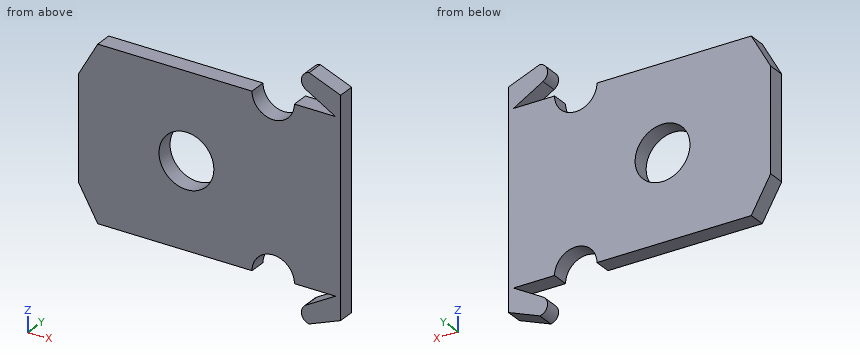
```python
from build123d import *

# Parameters (mm, degrees)
SKETCH1_R           = 0.8
BOSS_EXTRUDE1_DEPTH = 0.5


with BuildPart() as part:
    # Sketch1 → Boss-Extrude1 (new body)
    with BuildSketch(Plane(origin=(0, 0, 0), x_dir=(1, 0, 0), z_dir=(0, 1, 0))):
        with BuildLine():
            Line((0, 1.5), (0, -1.5))
            Line((0, -1.5), (0.566386859, -2.5))
            Line((0.566386859, -2.5), (5.066386859, -2.5))
            ThreePointArc((5.066386859, -2.5), (5.684410747, -1.881976112), (6.302434635, -2.5))
            Line((6.302434635, -2.5), (7.502434635, -2.5))
            Line((7.502434635, -2.5), (6.640167687, -3.000108496))
            ThreePointArc((6.640167687, -3.000108496), (6.510535737, -3.282386176), (6.733125956, -3.499039646))
            Line((6.733125956, -3.499039646), (7.651443218, -3.137476564))
            Line((7.651443218, -3.137476564), (7.651443218, 3.137476564))
            Line((7.651443218, 3.137476564), (6.733125956, 3.499039646))
            ThreePointArc((6.733125956, 3.499039646), (6.510535737, 3.282386176), (6.640167687, 3.000108496))
            Line((6.640167687, 3.000108496), (7.502434635, 2.5))
            Line((7.502434635, 2.5), (6.302434635, 2.5))
            ThreePointArc((6.302434635, 2.5), (5.684410747, 1.881976112), (5.066386859, 2.5))
            Line((5.066386859, 2.5), (0.566386859, 2.5))
            Line((0.566386859, 2.5), (0, 1.5))
        make_face()
        with Locations(Location((3.153366843, 0, 0), (0, 0, 270))):
            Circle(SKETCH1_R, mode=Mode.SUBTRACT)
    extrude(amount=BOSS_EXTRUDE1_DEPTH)


solid = part.part
```
Input: part model. Units: mm. Frame: model coordinates. Give positions to 0.01 mm unless a question says otherwise; leave off trailing zeros. Order: outer loops, then holes, each group sorted by start corner. A loop starts at its lowest first (then second) coordinate and runs counter-clockwise, first axis right, second up.
1. Cut plane B-B (x = 2.5). Return loops of the section in (y, z), and give its area (3 significant figures).
Computed:
outline: (0, -2.5) - (0.5, -2.5) - (0.5, -0.46) - (0, -0.46) - close; (0, 0.46) - (0.5, 0.46) - (0.5, 2.5) - (0, 2.5) - close
area: 2.04 mm2
2. Cut plane A-A (z = 0). Return loops of the section in (x, y).
Computed:
outline: (0, 0) - (2.35, 0) - (2.35, 0.5) - (0, 0.5) - close; (3.95, 0) - (7.65, 0) - (7.65, 0.5) - (3.95, 0.5) - close
3. Cut plane D-D (y = 0.3). Return loops of the section in (x, z), and give its area (3 significant figures).
Computed:
outline: (0, -1.5) - (0.57, -2.5) - (5.07, -2.5) arc R0.62 cw to (6.3, -2.5) - (7.5, -2.5) - (6.64, -3) arc R0.27 ccw to (6.73, -3.5) - (7.65, -3.14) - (7.65, 3.14) - (6.73, 3.5) arc R0.27 ccw to (6.64, 3) - (7.5, 2.5) - (6.3, 2.5) arc R0.62 cw to (5.07, 2.5) - (0.57, 2.5) - (0, 1.5) - close; hole circle Ø1.6 at (3.15, 0)
area: 35.8 mm2
4. Line query: probe 1 along X at (y, z) = (0.15, 0); probe 2 along Z at (x, y) = (6.75, 0.1); probe 3 along Z at (x, y) = (2.25, 0.05). Output: solid intervals per line, ascending.
Computed:
probe 1: x = 0 to 2.35, 3.95 to 7.65
probe 2: z = -3.49 to -2.94, -2.5 to 2.5, 2.94 to 3.49
probe 3: z = -2.5 to 2.5
5. Cut plane C-C (x = 7.25). Return loops of the section in (y, z).
Computed:
outline: (0, -3.3) - (0.5, -3.3) - (0.5, -2.65) - (0, -2.65) - close; (0, -2.5) - (0.5, -2.5) - (0.5, 2.5) - (0, 2.5) - close; (0, 2.65) - (0.5, 2.65) - (0.5, 3.3) - (0, 3.3) - close
